Geometry: final body of the model. Coordinates: model frame, mm. A direction names the side the tool comes from. Coordinates: 2 decimals unless noted, no trailing zeros. Loops run counter-clockwise (first coordinate to the right, second up) from the corner with the lowest first, then second, coordinate; pieces in that order, holes last. Notation, with made-up numbers: (-9, -25.5) - (45, -25.5) arc R18 cw to (45, -8.5) - close; hole circle Ø1 at (70.5, 12). An arc over 180 degrees is marked (long way). Write each question's results on one line, items separated by ' | '. Start each with the question number.
from build123d import *

# Parameters (mm, degrees)
BOSS_EXTRUDE1_START = -88.55
SKETCH1_W           = 43.6
SKETCH1_H           = 81.2
BOSS_EXTRUDE1_DEPTH = 11.55
BOSS_EXTRUDE2_START = 3.45
SKETCH2_W           = 20.55
SKETCH2_H           = 33
BOSS_EXTRUDE2_DEPTH = 7.45
BOSS_EXTRUDE3_START = 4.45
SKETCH3_W           = 6.3
SKETCH3_H           = 13
BOSS_EXTRUDE3_DEPTH = 6.45
BOSS_EXTRUDE4_START = 11.55
SKETCH4_W           = 26.85
SKETCH4_H           = 64.2
BOSS_EXTRUDE4_DEPTH = 1.05
BOSS_EXTRUDE5_START = -61.425
SKETCH5_W           = 32.8
SKETCH5_H           = 16.2
BOSS_EXTRUDE5_DEPTH = 10.275
BOSS_EXTRUDE6_START = -87.75
BOSS_EXTRUDE6_DEPTH = 12.35
BOSS_EXTRUDE7_START = -61.425
SKETCH7_W           = 32.8
SKETCH7_H           = 16.2
BOSS_EXTRUDE7_DEPTH = 10.275
BOSS_EXTRUDE8_START = -87.75
BOSS_EXTRUDE8_DEPTH = 12.35
CUT_EXTRUDE1_START  = -89.3
SKETCH9_W           = 43
SKETCH9_H           = 78
CUT_EXTRUDE1_DEPTH  = 10.8
CUT_EXTRUDE2_START  = 11.5
SKETCH10_R          = 1.45
CUT_EXTRUDE2_DEPTH  = 1.1
CUT_EXTRUDE3_START  = -88.45
CUT_EXTRUDE3_DEPTH  = 11.65
CUT_EXTRUDE4_START  = -59.775
SKETCH12_W          = 23.2
SKETCH12_H          = 13
CUT_EXTRUDE4_DEPTH  = 8.625
CUT_EXTRUDE5_START  = -52.65
SKETCH13_R          = 1.5
CUT_EXTRUDE5_DEPTH  = 1.5
CUT_EXTRUDE6_START  = -52.65
SKETCH14_W          = 2.15
SKETCH14_H          = 3
CUT_EXTRUDE6_DEPTH  = 1.5
CUT_EXTRUDE7_START  = -52.65
SKETCH15_R          = 1.5
CUT_EXTRUDE7_DEPTH  = 1.5
CUT_EXTRUDE8_START  = -52.65
SKETCH16_W          = 2.15
SKETCH16_H          = 3
CUT_EXTRUDE8_DEPTH  = 1.5
CUT_EXTRUDE9_START  = -70.4
SKETCH17_R          = 3.15
CUT_EXTRUDE9_DEPTH  = 1.3
CUT_EXTRUDE10_START = 8.5
SKETCH18_W          = 6
SKETCH18_H          = 4.4
CUT_EXTRUDE10_DEPTH = 2.4
CUT_EXTRUDE11_START = 11.5
SKETCH19_W          = 6
SKETCH19_H          = 4.4
CUT_EXTRUDE11_DEPTH = 1.1
CUT_EXTRUDE12_START = -77.75
SKETCH20_R          = 5.5
CUT_EXTRUDE12_DEPTH = 0.75
CUT_EXTRUDE13_START = -88.45
CUT_EXTRUDE13_DEPTH = 11.65
CUT_EXTRUDE14_START = -59.775
SKETCH22_W          = 23.2
SKETCH22_H          = 13
CUT_EXTRUDE14_DEPTH = 8.625
CUT_EXTRUDE15_START = -52.65
SKETCH23_R          = 1.5
CUT_EXTRUDE15_DEPTH = 1.5
CUT_EXTRUDE16_START = -52.65
SKETCH24_W          = 2.15
SKETCH24_H          = 3
CUT_EXTRUDE16_DEPTH = 1.5
CUT_EXTRUDE17_START = -52.65
SKETCH25_R          = 1.5
CUT_EXTRUDE17_DEPTH = 1.5
CUT_EXTRUDE18_START = -52.65
SKETCH26_W          = 2.15
SKETCH26_H          = 3
CUT_EXTRUDE18_DEPTH = 1.5
CUT_EXTRUDE19_START = -70.4
SKETCH27_R          = 3.15
CUT_EXTRUDE19_DEPTH = 1.3
CUT_EXTRUDE20_START = 8.5
SKETCH28_W          = 6
SKETCH28_H          = 4.4
CUT_EXTRUDE20_DEPTH = 2.4
CUT_EXTRUDE21_START = 11.5
SKETCH29_W          = 6
SKETCH29_H          = 4.4
CUT_EXTRUDE21_DEPTH = 1.1
CUT_EXTRUDE22_START = -77.75
SKETCH30_R          = 5.5
CUT_EXTRUDE22_DEPTH = 0.75


with BuildPart() as part:
    # Sketch1 → Boss-Extrude1 (new, symmetric)
    with BuildSketch(Plane(origin=(0, 0, 0), x_dir=(0, 0, -1), z_dir=(1, 0, 0)).offset(BOSS_EXTRUDE1_START)):
        with Locations((9.2, 0)):
            Rectangle(SKETCH1_W, SKETCH1_H)
    extrude(amount=BOSS_EXTRUDE1_DEPTH, both=True)



with BuildPart() as body_2:
    # Sketch2 → Boss-Extrude2 (new, symmetric)
    with BuildSketch(Plane.XY.offset(BOSS_EXTRUDE2_START)):
        with Locations((-61.425, 0)):
            Rectangle(SKETCH2_W, SKETCH2_H)
    extrude(amount=BOSS_EXTRUDE2_DEPTH, both=True)


with BuildPart() as part_1:
    add(part.part)

    add(body_2.part)  # Boss-Extrude3 merges body 2
    # Sketch3 → Boss-Extrude3 (add, symmetric)
    with BuildSketch(Plane.XY.offset(BOSS_EXTRUDE3_START)):
        with Locations((-74.85, 0)):
            Rectangle(SKETCH3_W, SKETCH3_H)
    extrude(amount=BOSS_EXTRUDE3_DEPTH, both=True)

    # Sketch4 → Boss-Extrude4 (add, symmetric)
    with BuildSketch(Plane.XY.offset(BOSS_EXTRUDE4_START)):
        with Locations((-64.575, 0)):
            Rectangle(SKETCH4_W, SKETCH4_H)
    extrude(amount=BOSS_EXTRUDE4_DEPTH, both=True)

    # Sketch5 → Boss-Extrude5 (add, symmetric)
    with BuildSketch(Plane(origin=(0, 0, 0), x_dir=(0, 0, -1), z_dir=(1, 0, 0)).offset(BOSS_EXTRUDE5_START)):
        with Locations((5.5, 24)):
            Rectangle(SKETCH5_W, SKETCH5_H)
    extrude(amount=BOSS_EXTRUDE5_DEPTH, both=True)

    # Sketch6 → Boss-Extrude6 (add, symmetric)
    with BuildSketch(Plane(origin=(0, 0, 0), x_dir=(0, 0, -1), z_dir=(1, 0, 0)).offset(BOSS_EXTRUDE6_START)):
        Polygon((25, 40), (25, 45.5), (11.2, 45.5), (5.7, 40), align=None)
    extrude(amount=BOSS_EXTRUDE6_DEPTH, both=True)

    # Sketch7 → Boss-Extrude7 (add, symmetric)
    with BuildSketch(Plane(origin=(0, 0, 0), x_dir=(0, 0, -1), z_dir=(1, 0, 0)).offset(BOSS_EXTRUDE7_START)):
        with Locations((5.5, -24)):
            Rectangle(SKETCH7_W, SKETCH7_H)
    extrude(amount=BOSS_EXTRUDE7_DEPTH, both=True)

    # Sketch8 → Boss-Extrude8 (add, symmetric)
    with BuildSketch(Plane(origin=(0, 0, 0), x_dir=(0, 0, -1), z_dir=(1, 0, 0)).offset(BOSS_EXTRUDE8_START)):
        Polygon((25, -40), (25, -45.5), (11.2, -45.5), (5.7, -40), align=None)
    extrude(amount=BOSS_EXTRUDE8_DEPTH, both=True)

    # Sketch9 → Cut-Extrude1 (cut, symmetric)
    with BuildSketch(Plane(origin=(0, 0, 0), x_dir=(0, 0, -1), z_dir=(1, 0, 0)).offset(CUT_EXTRUDE1_START)):
        with Locations((10.5, 0)):
            Rectangle(SKETCH9_W, SKETCH9_H)
    extrude(amount=CUT_EXTRUDE1_DEPTH, both=True, mode=Mode.SUBTRACT)

    # Sketch10 → Cut-Extrude2 (cut, symmetric)
    with BuildSketch(Plane.XY.offset(CUT_EXTRUDE2_START)):
        with Locations((-94.5, -29)):
            Circle(SKETCH10_R)
        with Locations((-94.5, 29)):
            Circle(SKETCH10_R)
        with Locations((-55.5, -29)):
            Circle(SKETCH10_R)
        with Locations((-55.5, 29)):
            Circle(SKETCH10_R)
    extrude(amount=CUT_EXTRUDE2_DEPTH, both=True, mode=Mode.SUBTRACT)

    # Sketch11 → Cut-Extrude3 (cut, symmetric)
    with BuildSketch(Plane(origin=(0, 0, 0), x_dir=(0, 0, -1), z_dir=(1, 0, 0)).offset(CUT_EXTRUDE3_START)):
        Polygon((20.1, 45.5), (15.7, 45.5), (15.7, 43.75), (13.55, 41.6), (22.25, 41.6), (20.1, 43.75), align=None)
    extrude(amount=CUT_EXTRUDE3_DEPTH, both=True, mode=Mode.SUBTRACT)

    # Sketch12 → Cut-Extrude4 (cut, symmetric)
    with BuildSketch(Plane(origin=(0, 0, 0), x_dir=(0, 0, -1), z_dir=(1, 0, 0)).offset(CUT_EXTRUDE4_START)):
        with Locations((5.5, 24)):
            Rectangle(SKETCH12_W, SKETCH12_H)
    extrude(amount=CUT_EXTRUDE4_DEPTH, both=True, mode=Mode.SUBTRACT)

    # Sketch13 → Cut-Extrude5 (cut, symmetric)
    with BuildSketch(Plane(origin=(0, 0, 0), x_dir=(0, 0, -1), z_dir=(1, 0, 0)).offset(CUT_EXTRUDE5_START)):
        with Locations((19.25, 24)):
            Circle(SKETCH13_R)
    extrude(amount=CUT_EXTRUDE5_DEPTH, both=True, mode=Mode.SUBTRACT)

    # Sketch14 → Cut-Extrude6 (cut, symmetric)
    with BuildSketch(Plane(origin=(0, 0, 0), x_dir=(0, 0, -1), z_dir=(1, 0, 0)).offset(CUT_EXTRUDE6_START)):
        with Locations((18.175, 24)):
            Rectangle(SKETCH14_W, SKETCH14_H)
    extrude(amount=CUT_EXTRUDE6_DEPTH, both=True, mode=Mode.SUBTRACT)

    # Sketch15 → Cut-Extrude7 (cut, symmetric)
    with BuildSketch(Plane(origin=(0, 0, 0), x_dir=(0, 0, -1), z_dir=(1, 0, 0)).offset(CUT_EXTRUDE7_START)):
        with Locations((-8.25, 24)):
            Circle(SKETCH15_R)
    extrude(amount=CUT_EXTRUDE7_DEPTH, both=True, mode=Mode.SUBTRACT)

    # Sketch16 → Cut-Extrude8 (cut, symmetric)
    with BuildSketch(Plane(origin=(0, 0, 0), x_dir=(0, 0, -1), z_dir=(1, 0, 0)).offset(CUT_EXTRUDE8_START)):
        with Locations((-7.175, 24)):
            Rectangle(SKETCH16_W, SKETCH16_H)
    extrude(amount=CUT_EXTRUDE8_DEPTH, both=True, mode=Mode.SUBTRACT)

    # Sketch17 → Cut-Extrude9 (cut, symmetric)
    with BuildSketch(Plane(origin=(0, 0, 0), x_dir=(0, 0, -1), z_dir=(1, 0, 0)).offset(CUT_EXTRUDE9_START)):
        with Locations((0, 24)):
            Circle(SKETCH17_R)
    extrude(amount=CUT_EXTRUDE9_DEPTH, both=True, mode=Mode.SUBTRACT)

    # Sketch18 → Cut-Extrude10 (cut, symmetric)
    with BuildSketch(Plane.XY.offset(CUT_EXTRUDE10_START)):
        with Locations((-65.4, 24)):
            Rectangle(SKETCH18_W, SKETCH18_H)
    extrude(amount=CUT_EXTRUDE10_DEPTH, both=True, mode=Mode.SUBTRACT)

    # Sketch19 → Cut-Extrude11 (cut, symmetric)
    with BuildSketch(Plane.XY.offset(CUT_EXTRUDE11_START)):
        with Locations((-65.4, 24)):
            Rectangle(SKETCH19_W, SKETCH19_H)
    extrude(amount=CUT_EXTRUDE11_DEPTH, both=True, mode=Mode.SUBTRACT)

    # Sketch20 → Cut-Extrude12 (cut, symmetric)
    with BuildSketch(Plane(origin=(0, 0, 0), x_dir=(0, 0, -1), z_dir=(1, 0, 0)).offset(CUT_EXTRUDE12_START)):
        with Locations((0, 24)):
            Circle(SKETCH20_R)
    extrude(amount=CUT_EXTRUDE12_DEPTH, both=True, mode=Mode.SUBTRACT)

    # Sketch21 → Cut-Extrude13 (cut, symmetric)
    with BuildSketch(Plane(origin=(0, 0, 0), x_dir=(0, 0, -1), z_dir=(1, 0, 0)).offset(CUT_EXTRUDE13_START)):
        Polygon((20.1, -45.5), (15.7, -45.5), (15.7, -43.75), (13.55, -41.6), (22.25, -41.6), (20.1, -43.75), align=None)
    extrude(amount=CUT_EXTRUDE13_DEPTH, both=True, mode=Mode.SUBTRACT)

    # Sketch22 → Cut-Extrude14 (cut, symmetric)
    with BuildSketch(Plane(origin=(0, 0, 0), x_dir=(0, 0, -1), z_dir=(1, 0, 0)).offset(CUT_EXTRUDE14_START)):
        with Locations((5.5, -24)):
            Rectangle(SKETCH22_W, SKETCH22_H)
    extrude(amount=CUT_EXTRUDE14_DEPTH, both=True, mode=Mode.SUBTRACT)

    # Sketch23 → Cut-Extrude15 (cut, symmetric)
    with BuildSketch(Plane(origin=(0, 0, 0), x_dir=(0, 0, -1), z_dir=(1, 0, 0)).offset(CUT_EXTRUDE15_START)):
        with Locations((19.25, -24)):
            Circle(SKETCH23_R)
    extrude(amount=CUT_EXTRUDE15_DEPTH, both=True, mode=Mode.SUBTRACT)

    # Sketch24 → Cut-Extrude16 (cut, symmetric)
    with BuildSketch(Plane(origin=(0, 0, 0), x_dir=(0, 0, -1), z_dir=(1, 0, 0)).offset(CUT_EXTRUDE16_START)):
        with Locations((18.175, -24)):
            Rectangle(SKETCH24_W, SKETCH24_H)
    extrude(amount=CUT_EXTRUDE16_DEPTH, both=True, mode=Mode.SUBTRACT)

    # Sketch25 → Cut-Extrude17 (cut, symmetric)
    with BuildSketch(Plane(origin=(0, 0, 0), x_dir=(0, 0, -1), z_dir=(1, 0, 0)).offset(CUT_EXTRUDE17_START)):
        with Locations((-8.25, -24)):
            Circle(SKETCH25_R)
    extrude(amount=CUT_EXTRUDE17_DEPTH, both=True, mode=Mode.SUBTRACT)

    # Sketch26 → Cut-Extrude18 (cut, symmetric)
    with BuildSketch(Plane(origin=(0, 0, 0), x_dir=(0, 0, -1), z_dir=(1, 0, 0)).offset(CUT_EXTRUDE18_START)):
        with Locations((-7.175, -24)):
            Rectangle(SKETCH26_W, SKETCH26_H)
    extrude(amount=CUT_EXTRUDE18_DEPTH, both=True, mode=Mode.SUBTRACT)

    # Sketch27 → Cut-Extrude19 (cut, symmetric)
    with BuildSketch(Plane(origin=(0, 0, 0), x_dir=(0, 0, -1), z_dir=(1, 0, 0)).offset(CUT_EXTRUDE19_START)):
        with Locations((0, -24)):
            Circle(SKETCH27_R)
    extrude(amount=CUT_EXTRUDE19_DEPTH, both=True, mode=Mode.SUBTRACT)

    # Sketch28 → Cut-Extrude20 (cut, symmetric)
    with BuildSketch(Plane.XY.offset(CUT_EXTRUDE20_START)):
        with Locations((-65.4, -24)):
            Rectangle(SKETCH28_W, SKETCH28_H)
    extrude(amount=CUT_EXTRUDE20_DEPTH, both=True, mode=Mode.SUBTRACT)

    # Sketch29 → Cut-Extrude21 (cut, symmetric)
    with BuildSketch(Plane.XY.offset(CUT_EXTRUDE21_START)):
        with Locations((-65.4, -24)):
            Rectangle(SKETCH29_W, SKETCH29_H)
    extrude(amount=CUT_EXTRUDE21_DEPTH, both=True, mode=Mode.SUBTRACT)

    # Sketch30 → Cut-Extrude22 (cut, symmetric)
    with BuildSketch(Plane(origin=(0, 0, 0), x_dir=(0, 0, -1), z_dir=(1, 0, 0)).offset(CUT_EXTRUDE22_START)):
        with Locations((0, -24)):
            Circle(SKETCH30_R)
    extrude(amount=CUT_EXTRUDE22_DEPTH, both=True, mode=Mode.SUBTRACT)


solid = part_1.part
1) Section query D-D on x = -73. Output: boundary loops of the cut face in (y, z), and give its area (3 significant figures).
2) Section query C-C on y = 8. Output: boundary loops of the cut face in (x, z).
3) Pull-direction query (Y, two-part tool) for faces 6 (the flat face through (-75.4, 43, -17)), 7 (the flat face through (-88, 40.6, -28)), 8 (the flat face through (-60, -17.5, -5)); classes: released by +Y, released by -Y, zero draft, split by the parting line, or undercut.
4) Material intervals for line 1 (Y direction, x = -55.5, z = 10.85); line 2 (Y direction, x = -77.7, z = 0); line 3 (X direction, y = -25, z = 6.5), sorted ascending. Write a range as [from, to].
5) Pin query (flat end, axial travel): pin 1 Ø4 at (x, y) = (-56.5, 18.5) entering from -Z; pin 2 Ø3 at (x, y) = (-93.5, 21) entering from -Z; pin 3 Ø1.5 at (x, z) = (-70.5, -7.5) entering from +Y. Return the tip coordinate at first contact, or that it passes through.
6) Section query B-B on x = -55.5. Output: boundary loops of the cut face in (y, z).
7) Access query for faces 1 (the flat face through (-61, -15.9, -13)), 2 (the flat face through (-76.8, 44, -18)), 3 (the flat face through (-88, 45, -15.7)), 4 (the flat face through (-56, 29, 10.4)), 5 (the flat face through (-78.5, 1, -10)). Directions: +Z, -Z, +X, -X, +Y, -Y. A direction counts if a zero-diameter tool reaches every point of the face in a straight line with its end or side. Return the directions, or none.
8) Section query A-A on z = -10. Output: boundary loops of the cut face in (x, y), and give its area (3 significant figures).
Returned:
1) outline: (-32.1, 10.5) - (-6.5, 10.5) - (-6.5, -2) - (6.5, -2) - (6.5, 10.5) - (32.1, 10.5) - (32.1, 12.6) - (-32.1, 12.6) - close | area: 297 mm²
2) outline: (-100.1, 11) - (-78.5, 11) - (-78.5, -31) - (-77, -31) - (-77, 10.5) - (-71.7, 10.5) - (-71.7, -4) - (-51.15, -4) - (-51.15, 12.6) - (-100.1, 12.6) - close
3) face 6: zero draft | face 7: released by +Y | face 8: undercut
4) line 1: y = [-32.1, -30.45], [-27.55, 27.55], [30.45, 32.1] | line 2: y = [-40.6, -29.5], [-18.5, 18.5], [29.5, 40.6] | line 3: x = [-78.5, -77], [-71.7, -68.4], [-62.4, -54.15]
5) pin 1: stops at z = -21.9 | pin 2: stops at z = 11 | pin 3: stops at y = 32.1
6) outline: (-32.1, -21.9) - (-15.9, -21.9) - (-15.9, -4) - (15.9, -4) - (15.9, -21.9) - (32.1, -21.9) - (32.1, 12.6) - (30.45, 12.6) - (30.45, 10.4) - (27.55, 10.4) - (27.55, 12.6) - (-27.55, 12.6) - (-27.55, 10.4) - (-30.45, 10.4) - (-30.45, 12.6) - (-32.1, 12.6) - close; hole (-30.5, -17.1) - (-17.5, -17.1) - (-17.5, 6.1) - (-30.5, 6.1) - close; hole (17.5, -17.1) - (30.5, -17.1) - (30.5, 6.1) - (17.5, 6.1) - close
7) face 1: -Z, +X | face 2: -X | face 3: -X, +Y | face 4: +Z | face 5: -Z, -X
8) outline: (-100.1, -44.3) - (-75.4, -44.3) - (-75.4, -40) - (-77, -40) - (-77, 40) - (-75.4, 40) - (-75.4, 44.3) - (-100.1, 44.3) - (-100.1, 39) - (-78.5, 39) - (-78.5, -39) - (-100.1, -39) - close; (-71.7, -32.1) - (-51.15, -32.1) - (-51.15, -30.5) - (-68.4, -30.5) - (-68.4, -17.5) - (-51.15, -17.5) - (-51.15, -15.9) - (-71.7, -15.9) - close; (-71.7, 15.9) - (-51.15, 15.9) - (-51.15, 17.5) - (-68.4, 17.5) - (-68.4, 30.5) - (-51.15, 30.5) - (-51.15, 32.1) - (-71.7, 32.1) - close | area: 593 mm²
